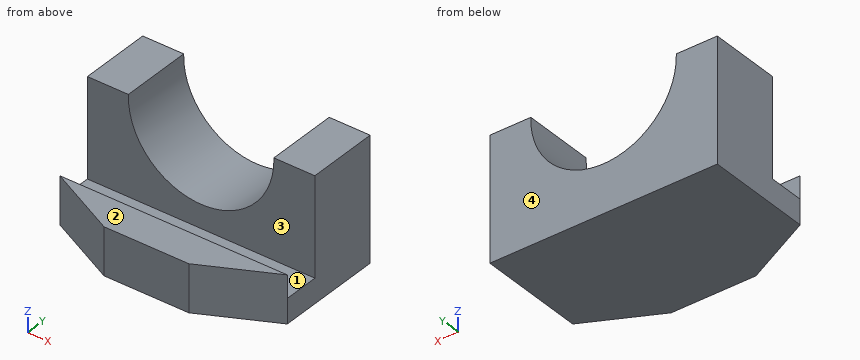
from build123d import *

# Parameters (mm, degrees)
F1_DEPTH      = 10
F1_DEPTH_BACK = 25
F3_DEPTH      = 111
F5_DEPTH      = 60.001


with BuildPart() as f1:
    # F0 (on Front) → F1 (new body, two sides)
    with BuildSketch(Plane.XZ) as f1_sk:
        with BuildLine():
            Line((0, 60), (0, 0))
            Line((0, 0), (111, 0))
            Line((111, 0), (111, 60))
            Line((111, 60), (91, 60))
            ThreePointArc((91, 60), (55.5, 23.341768), (20, 60))
            Line((20, 60), (0, 60))
        make_face()
    extrude(amount=F1_DEPTH)
    extrude(f1_sk.sketch, amount=-F1_DEPTH_BACK)

    # F2 (on Right) → F3 (join)
    with BuildSketch(Plane.YZ):
        Polygon((0, 12), (-10.259873, 12), (-27.44799, 12), (-27.44799, 23), (-44.633665, 23), (-44.633665, 0), (-27.168316, 0), (0, 0), align=None)
    extrude(amount=F3_DEPTH)

    # F4 (on Top) → F5 (cut, through all)
    with BuildSketch(Plane.XY):
        Polygon((111, -27.44799), (76.174157, -44.633665), (111, -44.633665), align=None)
        Polygon((34.825843, -44.633665), (0, -27.44799), (0, -44.633665), align=None)
    extrude(amount=F5_DEPTH, mode=Mode.SUBTRACT)


solid = f1.part
Build history of the part. All positions in model axes, mm. Face numbers are marked on the shaded views. Coordinates: 2 decimals unless noted, no trailing zeros. Order: outer loops, then holes, each group sorted by start corner. A loop starts at its lowest first (then second) coordinate and runs counter-clockwise, first axis right, second up. Notation, with made-up numbers: (46, 71) - (60, 71) arc R11 ccw to (60, 79) - close; hole circle Ø3 at (24, 36.5). An arc over 180 degrees is marked (long way). Write each question's results on one line, items separated by ' | '. Start each with the question number.
Item 1: Band-saw the part on B-B on x = 55.5. Write the cut outline in (y, z), and give its area (3 significant figures).
Item 2: Band-saw the part on D-D on z = 9. Write the cut outline in (x, y).
Item 3: Flat gauge pins, fed straight in: pin 1 (3 mm diameter, centred on x = 64, y = -27, fed in from +Z); pin 2 (8.5 mm diameter, centred on x = 57.5, y = -22.5, fed in from +Z). Where does each tip first touch, or does it go through?
Item 4: Band-saw the part on A-A on z = 38. Write the cut outline in (x, y), and give its area (3 significant figures).
Item 5: Wall check: probe 1 along Y at (x, z) = (95, 34.5); probe 2 along Z at (x, y) = (44, -30); probe 3 along Z at (x, y) = (90.5, -24.5). Give the ranges that are in metal, low to high. Write a range as [from, to].
Item 6: Mould opens along Y. For the marked faces 1, 2, 3 and 4 say: released by +Y, released by -Y, zero draft, split by the parting line, or undercut.
Item 7: Band-saw the part on C-C on y = 3. Write the cut outline in (x, z), and give its area (3 significant figures).
Numbers:
1) outline: (-44.63, 0) - (25, 0) - (25, 23.34) - (-10, 23.34) - (-10, 12) - (-27.45, 12) - (-27.45, 23) - (-44.63, 23) - close | area: 1,420 mm^2
2) outline: (0, -27.45) - (34.83, -44.63) - (76.17, -44.63) - (111, -27.45) - (111, 25) - (0, 25) - close
3) pin 1: z = 23 | pin 2: z = 12
4) outline: (0, -10) - (26.75, -10) - (26.75, 25) - (0, 25) - close; (84.25, -10) - (111, -10) - (111, 25) - (84.25, 25) - close | area: 1,870 mm^2
5) probe 1: [-10, 25] | probe 2: [0, 23] | probe 3: [0, 12]
6) face 1: undercut | face 2: zero draft | face 3: undercut | face 4: released by +Y
7) outline: (0, 0) - (111, 0) - (111, 60) - (91, 60) arc R35.52 cw (long way) to (20, 60) - (0, 60) - close | area: 4,600 mm^2
